Input: part model. Units: mm. Frame: model coordinates. A direction names the side the tool comes from. Coordinates: 2 decimals unless noted, no trailing zeros. Order: outer loops, then holes, each group sorted by start corner. A loop starts at its lowest first (then second) coordinate and runs counter-clockwise, first axis right, second up. Notation, with made-up numbers: (43.5, 55.25) - (87.5, 55.25) arc R17 ccw to (87.5, 83.25) - close; hole circle Ø11 at (66.5, 27.5). An arc over 180 degrees is marked (long way). Answer as CSV lines item,"result". Start each with the question number.
Item 1: Material intervals for line 1 along X through (y, z) = (-87, 127.5); line 2 along Z through (x, y) = (836.5, -111) (3 decimals); line 3 along Y through (x, z) = (70.5, -250.5), sorted ascending.
Item 2: First-contact query: pin 1 (1.5 mm diameter, centred on x = -646, z = -103, fed in from +Y); pin 2 (15 mm diameter, centred on x = -47, z = -278, fed in from +Y); pin 3 (2 mm diameter, centred on x = -693.5, z = 134.5, fed in from -Y). Flat tips, straight axial feed; report the tip coordinate or a pass-through.
Item 3: Section D-D (y = -219.5). Output: boundary loops of the cut face in (x, z) (1 decimal).
Item 4: Draft query along Y for faces 1 (the flat face through (-13, -104, -307.975)), 2 (the flat face through (-13, -444.5, 352)), 3 (the flat face through (-13, -342.9, 352)). Return one class per face: +Y half, -Y half, draft (parallel to the pull), parting line (faces both ways), or undercut.
Item 5: Access query for faces 4 (the flat face through (-13, -152.4, 39)), 5 (the flat face through (-13, -50.8, -282)), 6 (the flat face through (963.612, -244, 5)), 7 (the flat face through (-13, -393, 327.025)). Directions: +Z, -Z, +X, -X, +Y, -Y. A direction counts if a zero-diameter tool reaches every point of the face in a straight line with its end or side. Return the directions, or none.
Item 6: Section B-B (y = -69). Output: boundary loops of the cut face in (x, z) (1 decimal).
Item 7: Section C-C (z = 281). Output: boundary loops of the cut face in (x, y).
Item 8: Section A-A (x = -462). Output: boundary loops of the cut face in (y, z) (3 decimals), and give its area (3 significant figures).
from build123d import *

# Parameters (mm, degrees)
F0_W     = 12.7
F0_H     = 69.85
F0_H_2   = 50.8
F0_H_3   = 584.2
F1_DEPTH = 495.3
F0_W_2   = 1927.225
F2_DEPTH = 152.4
F3_DEPTH = 158.75
F4_DEPTH = 495.3
F5_DEPTH = 50.8
F6_W     = 101.6
F6_H     = 50.8
F7_DEPTH = 1952.625
F8_DEPTH = 152.4


with BuildPart() as f1:
    # F0 (on Front) → F1 (new body)
    with BuildSketch(Plane.XZ):
        with Locations((-969.9625, -342.9)):
            Rectangle(F0_W, F0_H)
        with Locations((-969.9625, -282.575)):
            Rectangle(F0_W, F0_H_2)
        with Locations((-969.9625, 34.925)):
            Rectangle(F0_W, F0_H_3)
        with Locations((-969.9625, 352.425)):
            Rectangle(F0_W, F0_H_2)
    extrude(amount=F1_DEPTH)

    # F0 (on Front) → F2 (join)
    with BuildSketch(Plane.XZ):
        with Locations((0, 352.425)):
            Rectangle(F0_W_2, F0_H_2)
        with Locations((0, -282.575)):
            Rectangle(F0_W_2, F0_H_2)
    extrude(amount=F2_DEPTH)

    # F0 (on Front) → F3 (join)
    with BuildSketch(Plane.XZ):
        with Locations((0, 34.925)):
            Rectangle(F0_W_2, F0_H_3)
        with Locations((0, 352.425)):
            Rectangle(F0_W_2, F0_H_2)
        with Locations((0, -282.575)):
            Rectangle(F0_W_2, F0_H_2)
    extrude(amount=F3_DEPTH)

    # F0 (on Front) → F4 (join)
    with BuildSketch(Plane.XZ):
        with Locations((969.9625, 34.925)):
            Rectangle(F0_W, F0_H_3)
        with Locations((969.9625, 352.425)):
            Rectangle(F0_W, F0_H_2)
        with Locations((969.9625, -282.575)):
            Rectangle(F0_W, F0_H_2)
        with Locations((969.9625, -342.9)):
            Rectangle(F0_W, F0_H)
    extrude(amount=F4_DEPTH)

    # F0 (on Front) → F5 (cut)
    with BuildSketch(Plane.XZ):
        with Locations((0, 352.425)):
            Rectangle(F0_W_2, F0_H_2)
        with Locations((0, -282.575)):
            Rectangle(F0_W_2, F0_H_2)
    extrude(amount=F5_DEPTH, mode=Mode.SUBTRACT)

    # F6 (on face) → F7 (join, through all)
    with BuildSketch(Plane(origin=(-976.3125, 0, 0), x_dir=(0, -1, 0), z_dir=(-1, 0, 0))):
        with Locations((393.7, 352.425)):
            Rectangle(F6_W, F6_H)
    extrude(amount=-F7_DEPTH)

    # F0 (on Front) → F8 (cut)
    with BuildSketch(Plane.XZ):
        with Locations((0, 34.925)):
            Rectangle(F0_W_2, F0_H_3)
    extrude(amount=F8_DEPTH, mode=Mode.SUBTRACT)


solid = f1.part
Determined:
1,line 1,"x = -976.31 to -963.61, 963.61 to 976.31"
1,line 2,"z = -307.975 to -257.175, 327.025 to 377.825"
1,line 3,"y = -158.75 to -152.4"
2,pin 1,"stops at y = -152.4"
2,pin 2,"stops at y = -50.8"
2,pin 3,"stops at y = -158.75"
3,outline,"(-976.3, -377.8) - (-963.6, -377.8) - (-963.6, 377.8) - (-976.3, 377.8) - close; (963.6, -377.8) - (976.3, -377.8) - (976.3, 377.8) - (963.6, 377.8) - close"
4,face 1,"draft"
4,face 2,"-Y half"
4,face 3,"undercut"
5,face 4,"+Y"
5,face 5,"+Z, -Z, +Y"
5,face 6,"none"
5,face 7,"-Z, -Y"
6,outline,"(-976.3, -377.8) - (-963.6, -377.8) - (-963.6, -308) - (963.6, -308) - (963.6, -377.8) - (976.3, -377.8) - (976.3, 377.8) - (-976.3, 377.8) - close; hole (-963.6, -257.2) - (963.6, -257.2) - (963.6, 327) - (-963.6, 327) - close"
7,outline,"(-976.31, -495.3) - (-963.61, -495.3) - (-963.61, -158.75) - (963.61, -158.75) - (963.61, -495.3) - (976.31, -495.3) - (976.31, 0) - (963.61, 0) - (963.61, -152.4) - (-963.61, -152.4) - (-963.61, 0) - (-976.31, 0) - close"
8,outline,"(-444.5, 327.025) - (-342.9, 327.025) - (-342.9, 377.825) - (-444.5, 377.825) - close; (-158.75, -307.975) - (-50.8, -307.975) - (-50.8, -257.175) - (-152.4, -257.175) - (-152.4, 327.025) - (-50.8, 327.025) - (-50.8, 377.825) - (-158.75, 377.825) - close"
8,area,"19,800 mm^2"
